```python
from build123d import *

# Parameters (mm, degrees)
SKETCH1_W           = 1000
SKETCH1_H           = 500
BOSS_EXTRUDE1_DEPTH = 15
SKETCH2_W           = 15
SKETCH2_H           = 499.509580663
BOSS_EXTRUDE2_DEPTH = 800
BOSS_EXTRUDE3_REACH = 987
SKETCH3_W           = 459.509580663
SKETCH3_H           = 15
SKETCH4_R           = 20
CUT_EXTRUDE1_DEPTH  = 816


with BuildPart() as part:
    # Sketch1 → Boss-Extrude1 (new body)
    with BuildSketch(Plane(origin=(0, 0, 0), x_dir=(1, 0, 0), z_dir=(0, 1, 0))):
        Rectangle(SKETCH1_W, SKETCH1_H)
    extrude(amount=BOSS_EXTRUDE1_DEPTH)

    # Sketch2 → Boss-Extrude2 (add)
    with BuildSketch(Plane.XZ):
        with Locations((-492.5, 0.245209669)):
            Rectangle(SKETCH2_W, SKETCH2_H)
        with Locations((492.5, 0.245209669)):
            Rectangle(SKETCH2_W, SKETCH2_H)
    extrude(amount=BOSS_EXTRUDE2_DEPTH)

    # Sketch3 → Boss-Extrude3 (add, up to next)
    with BuildSketch(Plane(origin=(-485, 0, 0), x_dir=(0, 0, -1), z_dir=(1, 0, 0)), mode=Mode.PRIVATE) as boss_extrude3_sk1:
        with Locations((-0.245209669, -77.5)):
            Rectangle(SKETCH3_W, SKETCH3_H)
    boss_extrude3_tool1 = extrude(boss_extrude3_sk1.sketch, amount=BOSS_EXTRUDE3_REACH, mode=Mode.PRIVATE) - part.part
    add(boss_extrude3_tool1.solids().sort_by_distance((-485, -77.5, 0.24521))[0])

    # Sketch4 → Cut-Extrude1 (cut, through all)
    with BuildSketch(Plane(origin=(0, 15, 0), x_dir=(1, 0, 0), z_dir=(0, 1, 0))):
        with Locations((-420, 250)):
            Circle(SKETCH4_R)
    extrude(amount=-CUT_EXTRUDE1_DEPTH, mode=Mode.SUBTRACT)


solid = part.part
```
Part model, mm, in its own coordinate system. A direction names the side the tool comes from. Round coordinates to 2 decimals unless told otherwise and drop trailing zeros. Order: outer loops, then holes, each group sorted by start corner. A loop starts at its lowest first (then second) coordinate and runs counter-clockwise, first axis right, second up. Notation, with made-up numbers: M 82,77 L 111,77 A18 ccw 111,86 Z; hole C 61,26.25 d3. An arc over 180 degrees is marked long. Put each result on its own line as item: value. Start each with the question number.
1. Slice it at A-A on y = -520. List the corners of the cut face in (x, z).
2. Slice it at B-B on x = 79. List the corners of the cut face in (y, z), then the cut area to 3 significant figures.
3. Tool access for faces 4 (the face through (500, -398, 4)), 5 (the face through (-7, 0, -3)): list every direction of +Z, -Z, +X, -X, +Y, -Y with a clear straight run to the whole face (end or side of a thin tool).
4. Drop flat-ended pins along their axis: pin 1 (12 mm diameter, centred on x = -222, y = -74.5, fed in from -Z); pin 2 (1 mm diameter, centred on x = -150.5, z = 171.5, fed in from -Y); pin 3 (12 mm diameter, centred on x = -491, y = -536, fed in from -Z). Give the stop position or say it passes through.
5. Drill centre lines: probe 1 along X at (y, z) = (-639.5, 155); probe 2 along Y at (x, z) = (-95.5, -55.5). Where is each one in solid material? Low to high. Write a range as [from, to].
6. Two-plate mould, pull along Y, no slides. Class faces 1 (the face through (-7, 15, -4)), 2 (the face through (-7, -70, 3)), 3 (the face through (-7, -85, 3)): +Y half, -Y half, draft (parallel to the pull), parting line (faces both ways), or undercut.
7. Slice it at C-C on z = -42. List the corners of the cut face in (x, y).
Findings:
1. outline: M -500,-249.51 L -485,-249.51 L -485,250 L -500,250 Z; M 485,-249.51 L 500,-249.51 L 500,250 L 485,250 Z
2. outline: M -85,-229.51 L -70,-229.51 L -70,230 L -85,230 Z; M 0,-250 L 15,-250 L 15,250 L 0,250 Z
2. area: 14,400 mm2
3. face 4: +Z, -Z, +X, +Y, -Y
3. face 5: +Z, -Z
4. pin 1: z = -229.51
4. pin 2: y = -85
4. pin 3: z = -249.51
5. probe 1: [-500, -485], [485, 500]
5. probe 2: [-85, -70], [0, 15]
6. face 1: +Y half
6. face 2: undercut
6. face 3: -Y half
7. outline: M -500,-800 L -485,-800 L -485,-85 L 485,-85 L 485,-800 L 500,-800 L 500,15 L -500,15 Z; hole M -485,-70 L 485,-70 L 485,0 L -485,0 Z
